Autodesk Inventor part; units mm, degrees
ref_plane "YZ Plane" through (0, 0, 0) normal (1, 0, 0) x (0, 1, 0)
ref_plane "XZ Plane" through (0, 0, 0) normal (0, 1, 0) x (-1, 0, 0)
ref_plane "XY Plane" through (0, 0, 0) normal (0, 0, 1) x (1, 0, 0)
sketch "Sketch1" plane through (0, 0, 0) normal (0, 1, 0) x (-1, 0, 0)
  line L0 (0, 0) -> (167.4876, 0)
  line L1 (167.4876, 0) -> (167.4876, -27)
  line L2 (167.4876, -27) -> (0, -27)
  line L3 (0, -27) -> (0, 0)
  dimension "d0" = 167.4876
  dimension "d1" = 27
extrude "Extrusion1" add sketch "Sketch1" along normal blind 2.54
sketch "Sketch2" plane through (0, 2.54, 0) normal (0, 1, 0) x (1, 0, 0)
  circle A0 centre (-45, 13.5001) radius 2.5
  line L0 (-167.4876, 0) -> (0, 0)
  line L1 (0, 0) -> (0, 27)
  circle A1 centre (-145, 13.5128) radius 2.5
  dimension "d4" = 5
  dimension "d5" = 13.5001
  dimension "d6" = 45
  dimension "d7" = 5
  dimension "d8" = 13.5128
  dimension "d9" = 100
extrude "Extrusion2" add sketch "Sketch2" along normal blind 17.5
properties part number "DinRail"
Read the model definition and answer for the solid it produces. Units are mm, in the model's axes. A direction names the side the tool comes from. Give positions to 0.01 mm unless a question says otherwise; leave off trailing zeros. Write each loop counter-clockwise with the first axis right and the second up, starting at its lowest first coordinate (ties: lowest second). Pieces come first, ordered by that corner, then holes. Notation, with made-up numbers: M 19.5,71 L 55.5,71 A23 cw 55.5,79 Z; hole C 68.25,17.25 d8. An arc over 180 degrees is marked long. Put each result on its own line as item: value. Start each with the question number.
1. For a pull along X with two mould halves and no side action, classify faces 3 (the cylindrical face through (-42.615, 11.168, -12.749)), 4 (the flat face through (-145, 20.04, -14)) as released by +X, released by -X, zero draft, split by the parting line, or undercut.
2. Consider line 1 along X through (y, z) = (13.5, -13.75); line 2 along Y through (x, z) = (-17, -15); line 3 along X through (y, z) = (3.75, -15.5). Determine where each line is inside the solid, lowest interval first.
3. Which of the six approach directions +Z, -Z, +X, -X, +Y, -Y give full straight-line access (tool end or side, diameter ignored) to faces 1 (the cylindrical face through (-142.615, 11.168, -12.762)), 2 (the flat face through (-83, 0, -13))?
4. The part is cut by section C-C, the plane y = 4.5. Give the vertices of the cut face in (x, z).
5. Each of these flat-tipped pins is pushed along its axis until it touches: pin 1 Ø8 at (x, z) = (-144, -16) entering from -Y; pin 2 Ø2 at (x, y) = (-44.5, 7.5) entering from +Z. Where does it stop, or does it pass through?
6. The part is cut by section A-A, the plane x = -45. Give the vertices of the cut face in (y, z), and give its area (3 significant figures).
7. The part is cut by section D-D, the plane x = -102. Give the vertices of the cut face in (y, z), and give its area (3 significant figures).
8. The part is cut by section B-B, the plane z = -5.75. Give the vertices of the cut face in (x, y), and give its area (3 significant figures).
Final values:
1. face 3: undercut
1. face 4: zero draft
2. line 1: x = -147.49 to -142.51, -47.49 to -42.51
2. line 2: y = 0 to 2.54
2. line 3: x = -146.52 to -143.48, -46.5 to -43.5
3. face 1: +Y
3. face 2: +Z, -Z, +X, -X, -Y
4. outline: C -145,-13.51 d5; C -45,-13.5 d5
5. pin 1: stops at y = 0
5. pin 2: stops at z = -11
6. outline: M 0,-27 L 2.54,-27 L 2.54,-16 L 20.04,-16 L 20.04,-11 L 2.54,-11 L 2.54,0 L 0,0 Z
6. area: 156 mm²
7. outline: M 0,-27 L 2.54,-27 L 2.54,0 L 0,0 Z
7. area: 68.6 mm²
8. outline: M -167.49,0 L 0,0 L 0,2.54 L -167.49,2.54 Z
8. area: 425 mm²
